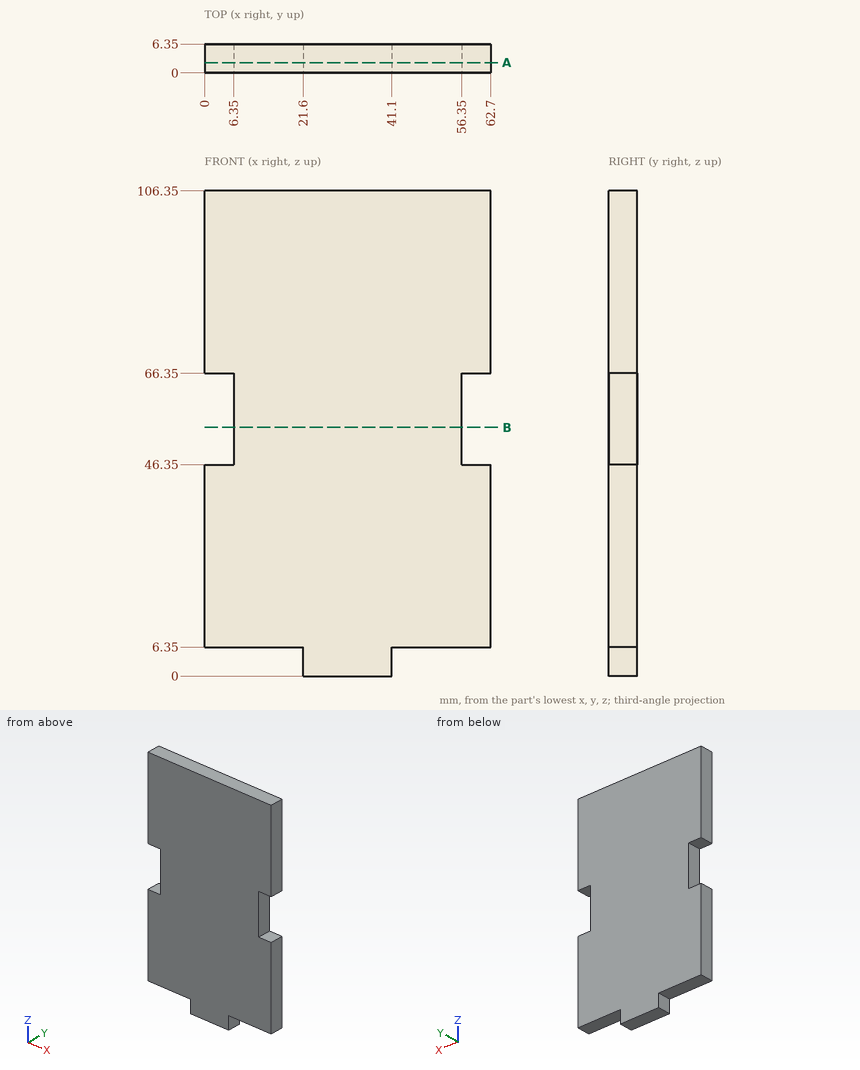
Print and shaded views of the part. All mm, measured from the part's lowest x, y and z. Round coordinates to 2 decimals unless told otherwise and drop trailing zeros. Write each loop counter-clockwise with the first axis right and the second up, starting at its lowest first coordinate (ties: lowest second). Pieces come first, ordered by that corner, then holes.
(1) Slice it at A-A, the plane y = 2.25. Write the cut outline in (x, z), and give its area (3 significant figures).
(2) Drop flat-ended pins along their axis: P1, Ø1, axis at x = 46.5, y = 2, coming from the -Z side; P2, Ø1.9, axis at y = 3, z = 4.5, coming from the +X side; P3, Ø1.9, axis at y = 3.5, z = 56, coming from the -X side. Give the stop position or say it passes through.
(3) Probe line 1 along Z through (x, y) = (49, 1.5); line 2 along X through (y, z) = (5.5, 56.5); line 3 along X through (y, z) = (5.5, 5.5). List the from-to ranges inside material, lowest first.
(4) Slice it at B-B, the plane z = 54.5. Write the cut outline in (x, y).
From the geometry:
1. outline: (0, 6.35) - (21.6, 6.35) - (21.6, 0) - (41.1, 0) - (41.1, 6.35) - (62.7, 6.35) - (62.7, 46.35) - (56.35, 46.35) - (56.35, 66.35) - (62.7, 66.35) - (62.7, 106.35) - (0, 106.35) - (0, 66.35) - (6.35, 66.35) - (6.35, 46.35) - (0, 46.35) - close
1. area: 6,140 mm2
2. P1: stops at z = 6.35
2. P2: stops at x = 41.1
2. P3: stops at x = 6.35
3. line 1: z = 6.35 to 106.35
3. line 2: x = 6.35 to 56.35
3. line 3: x = 21.6 to 41.1
4. outline: (6.35, 0) - (56.35, 0) - (56.35, 6.35) - (6.35, 6.35) - close
